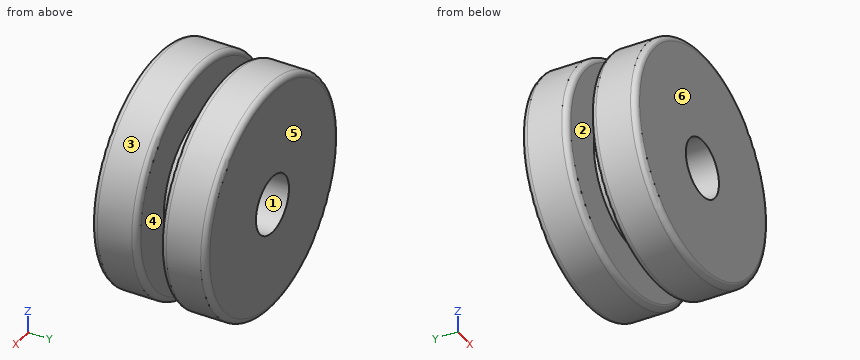
```python
from build123d import *

# Parameters (mm, degrees)
F0_R     = 100
F1_DEPTH = 40
F2_R     = 60
F3_DEPTH = 20
F4_R     = 100
F5_DEPTH = 40
F6_R     = 25
F7_DEPTH = 100
F8_R     = 5


with BuildPart() as f1:
    # F0 (on Front) → F1 (new body)
    with BuildSketch(Plane.XZ):
        Circle(F0_R)
    extrude(amount=F1_DEPTH)

    # F2 (on face) → F3 (join)
    with BuildSketch(Plane.XZ.offset(40)):
        Circle(F2_R)
    extrude(amount=F3_DEPTH)

    # F4 (on face) → F5 (join)
    with BuildSketch(Plane.XZ.offset(60)):
        Circle(F4_R)
    extrude(amount=F5_DEPTH)

    # F6 (on face) → F7 (cut)
    with BuildSketch(Plane.XZ.offset(100)):
        with Locations((0, -5.704428)):
            Circle(F6_R)
    extrude(amount=-F7_DEPTH, mode=Mode.SUBTRACT)

    # F8
    f8_edges = [f1.edges().sort_by_distance(p)[0] for p in [
        (-100, -100, 0),
        (-100, -60, 0),
        (-100, -40, 0),
        (-100, 0, 0),
    ]]
    fillet(f8_edges, radius=F8_R)


solid = f1.part
```
The model under review builds one solid part; all positions refer to its coordinate system, in mm. Face numbers are marked on the shaded views. A direction names the side the tool comes from. Give positions to 0.01 mm unless a question says otherwise; leave off trailing zeros. Write each loop counter-clockwise with the first axis right and the second up, starting at its lowest first coordinate (ties: lowest second). Pieces come first, ordered by that corner, then holes. Notation, with made-up numbers: M 21,52.25 L 39,52.25 A27 cw 39,86.25 Z; hole C -7.5,-37 d10. An arc over 180 degrees is marked long. Write item = value, one per line. Start each with the question number.
Q1. Mouldability with a two-part tool opening along Y and no side actions: class the marked faces 3, 4, 5 and 6 as released by +Y, released by -Y, zero draft, split by the parting line, or undercut.
Q2. For line 1 (Z direction, x = 0, y = -55); line 2 (Z direction, x = 0, y = -22); line 3 (Y direction, x = -43.5, z = -57), list the stretches that pass through material, from the lowest coordinate up.
Q3. We need section A-A (x = 0). State the section outline as (y, z) points, plus the area to 3 significant figures.
Q4. We need section D-D (y = -9.5). State the section outline as (x, z) points, plus the area to 3 significant figures.
Q5. Machinability: for the marked faces 1 and 2, which of the approach directions +Z, -Z, +X, -X, +Y, -Y give a long, thin tool a straight path to every point of the face, cutting with its end or side? Answer none if there is none.
Q6. Clearance check with flat-ended pins moving along their axes: pin 1 (1 mm diameter, centred on y = -75.5, z = 26.5, fed in from -X); pin 2 (12 mm diameter, centred on x = -30.5, y = -62, fed in from -Z); pin 3 (1.5 mm diameter, centred on x = -13, y = -16.5, fed in from +Z). State where each tip first meets the part, or that it passes through.
Q7. We need section B-B (z = 0). State the section outline as (x, y) points.
Q8. We need section C-C (y = -50.5). State the section outline as (x, z) points.
Result set:
q1.face_3 = zero draft
q1.face_4 = undercut
q1.face_5 = released by +Y
q1.face_6 = released by -Y
q2.line_1 = -60 to -30.7, 19.3 to 60
q2.line_2 = -100 to -30.7, 19.3 to 100
q2.line_3 = -100 to -60, -40 to 0
q3.outline = M -100,-95 A5 ccw -95,-100 L -65,-100 A5 ccw -60,-95 L -60,-60 L -40,-60 L -40,-95 A5 ccw -35,-100 L -5,-100 A5 ccw 0,-95 L 0,-30.7 L -100,-30.7 Z; M -100,19.3 L 0,19.3 L 0,95 A5 ccw -5,100 L -35,100 A5 ccw -40,95 L -40,60 L -60,60 L -60,95 A5 ccw -65,100 L -95,100 A5 ccw -100,95 Z
q3.area = 13,400 mm2
q4.outline = C 0,0 d200; hole C 0,-5.7 d50
q4.area = 29,500 mm2
q5.face_1 = +Y, -Y
q5.face_2 = none
q6.pin_1 = -96.56
q6.pin_2 = -96.79
q6.pin_3 = 99.25
q7.outline = M -100,-95 A5 ccw -95,-100 L -24.34,-100 L -24.34,0 L -95,0 A5 ccw -100,-5 L -100,-35 A5 ccw -95,-40 L -60,-40 L -60,-60 L -95,-60 A5 ccw -100,-65 Z; M 24.34,-100 L 95,-100 A5 ccw 100,-95 L 100,-65 A5 ccw 95,-60 L 60,-60 L 60,-40 L 95,-40 A5 ccw 100,-35 L 100,-5 A5 ccw 95,0 L 24.34,0 Z
q8.outline = C 0,0 d120; hole C 0,-5.7 d50
